```python
from build123d import *

# Parameters (mm, degrees)
F1_DEPTH = 4
F2_R     = 1.5
F3_DEPTH = 50


with BuildPart() as f1:
    # F0 (on Front) → F1 (new body)
    with BuildSketch(Plane.XZ):
        with BuildLine():
            Line((23.162254, 10.430464), (-28.377483, 10.430464))
            ThreePointArc((-28.377483, 10.430464), (-31.913017, 8.965997), (-33.377483, 5.430464))
            Line((-33.377483, 5.430464), (-33.377483, -3.344371))
            ThreePointArc((-33.377483, -3.344371), (-31.913017, -6.879905), (-28.377483, -8.344371))
            Line((-28.377483, -8.344371), (23.162254, -8.344371))
            ThreePointArc((23.162254, -8.344371), (26.697788, -6.879905), (28.162254, -3.344371))
            Line((28.162254, -3.344371), (28.162254, 5.430464))
            ThreePointArc((28.162254, 5.430464), (26.697788, 8.965997), (23.162254, 10.430464))
        make_face()
    extrude(amount=F1_DEPTH)

    # F2 (on face) → F3 (join)
    with BuildSketch(Plane.YZ.offset(28.162254)):
        with Locations((-1.518368, 1.043046)):
            Circle(F2_R)
    extrude(amount=F3_DEPTH)


solid = f1.part
```
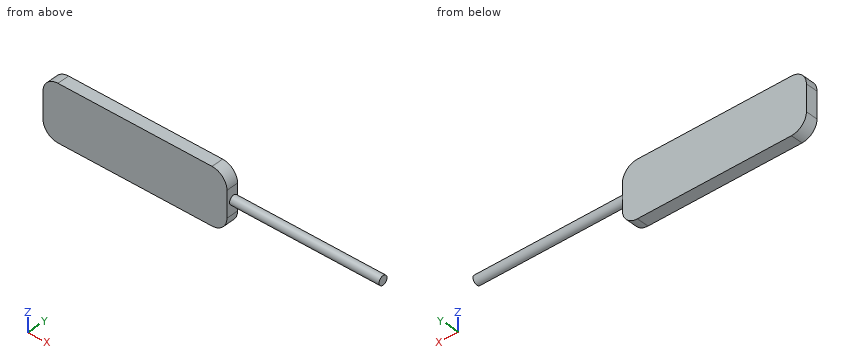
Work out the finished part from the listing and answer in its coordinate system (mm). Coordinates: 2 decimals unless noted, no trailing zeros. Write each loop counter-clockwise with the first axis right and the second up, starting at its lowest first coordinate (ties: lowest second). Pieces come first, ordered by that corner, then holes.
Q1. A cutting plane is placed at A-A, the plane y = -1.85. Give the vertices of the cut face in (x, z), then the cut area to 3 significant figures.
Q2. Each of these flat-tipped pins is pushed along its axis until it touches: pin 1 Ø2 at (x, y) = (66, -0.5) entering from -Z; pin 2 Ø1 at (y, z) = (-1.5, -4) entering from -X; pin 3 Ø3 at (x, z) = (-8, 7.5) entering from +Y; pin 4 Ø5 at (x, z) = (52, 1) entering from -Y. Where does it stop, or does it pass through?
Q3. A cutting plane is placed at D-D, the plane z = -6.25. Give the vertices of the cut face in (x, y), then the cut area to 3 significant figures.
Q4. A cutting plane is placed at C-C, the plane x = 41. Give the vertices of the cut face in (y, z).
Q5. A cutting plane is placed at B-B, the plane z = 4. Give the vertices of the cut face in (x, y), then the cut area to 3 significant figures.
Q6. Find the intervals of material crossed by line 1 (X direction, y = -0.9, z = -0.5); line 2 (X direction, y = -1.65, z = -4); line 3 (Z direction, x = 43, y = -2.75), in increasing order.
Findings below:
1. outline: (-33.38, -3.34) arc R5 ccw to (-28.38, -8.34) - (23.16, -8.34) arc R5 ccw to (28.16, -3.34) - (28.16, -0.42) - (78.16, -0.42) - (78.16, 2.51) - (28.16, 2.51) - (28.16, 5.43) arc R5 ccw to (23.16, 10.43) - (-28.38, 10.43) arc R5 ccw to (-33.38, 5.43) - close
1. area: 1,280 mm2
2. pin 1: stops at z = -0.46
2. pin 2: stops at x = -33.38
2. pin 3: stops at y = 0
2. pin 4: stops at y = -3.02
3. outline: (-32.45, -4) - (27.23, -4) - (27.23, 0) - (-32.45, 0) - close
3. area: 239 mm2
4. outline: circle Ø3 at (-1.52, 1.04)
5. outline: (-33.38, -4) - (28.16, -4) - (28.16, 0) - (-33.38, 0) - close
5. area: 246 mm2
6. line 1: x = -33.38 to 28.16
6. line 2: x = -33.33 to 28.12
6. line 3: z = 0.19 to 1.9
